```python
from build123d import *

# Parameters (mm, degrees)
F1_DEPTH  = 63.5
F0_W      = 25.4
F0_H      = 5.545384808
F0_H_2    = 19.05
F0_H_3    = 3.979615192
F2_DEPTH  = 17.526
F3_DEPTH  = 25.4
F4_DEPTH  = 7.9375
F4_FACE_W = 68.3895
F4_FACE_H = 28.575
F6_R      = 6.35


with BuildPart() as f1:
    # F0 (on Front) → F1 (new body, symmetric)
    with BuildSketch(Plane.XZ):
        Polygon((-41.275, -9.525), (41.275, -9.525), (41.275, 9.525), (22.225, 9.525), (-41.275, 9.525), align=None)
    extrude(amount=F1_DEPTH, both=True)

    # F0 (on Front) → F2 (join, symmetric)
    with BuildSketch(Plane.XZ):
        Polygon((-41.275, -9.525), (41.275, -9.525), (41.275, 9.525), (22.225, 9.525), (-41.275, 9.525), align=None)
        with BuildLine():
            Line((22.225, 9.525), (41.275, 9.525))
            Line((41.275, 9.525), (41.275, 28.8728918047))
            ThreePointArc((41.275, 28.8728918047), (44.1836383767, 35.8949660218), (51.2057125939, 38.8036043985))
            Line((51.2057125939, 38.8036043985), (60.325, 38.8036043985))
            Line((60.325, 38.8036043985), (60.325, 57.8536043985))
            Line((60.325, 57.8536043985), (51.2057125939, 57.8536043985))
            ThreePointArc((51.2057125939, 57.8536043985), (30.7132541951, 49.3653502034), (22.225, 28.8728918047))
            Line((22.225, 28.8728918047), (22.225, 9.525))
        make_face()
        with BuildLine():
            add(Edge.make_bspline(
                [(-41.275, 9.525), (-35.7294939458, 54.0499053895), (8.4615461528, 64.4009560347), (60.325, 63.3989892066)],
                knots=[0, 0, 0, 0, 114.9998552739, 114.9998552739, 114.9998552739, 114.9998552739], degree=3))
            Line((-41.275, 9.525), (22.225, 9.525))
            Line((22.225, 9.525), (22.225, 28.8728918047))
            ThreePointArc((22.225, 28.8728918047), (30.7132541951, 49.3653502034), (51.2057125939, 57.8536043985))
            Line((51.2057125939, 57.8536043985), (60.325, 57.8536043985))
            Line((60.325, 57.8536043985), (60.325, 63.3989892066))
        make_face()
        with Locations((73.025, 60.6262968025)):
            Rectangle(F0_W, F0_H)
        Polygon((111.125, 63.3989892066), (85.725, 63.3989892066), (85.725, 57.8536043985), (85.725, 38.8036043985), (85.725, 34.8239892066), (111.125, 34.8239892066), align=None)
        with Locations((73.025, 48.3286043985)):
            Rectangle(F0_W, F0_H_2)
        with Locations((73.025, 36.8137968025)):
            Rectangle(F0_W, F0_H_3)
    extrude(amount=F2_DEPTH, both=True)

    # F3 (add, symmetric): a face of the model
    f3_faces = [f1.faces().sort_by_distance(p)[0] for p in [
        (31.3502124895, -17.526, 38.5126856462),
    ]]
    extrude(f3_faces, amount=F3_DEPTH, both=True)

    # F4 (add, symmetric): a face of the model
    f4_faces = [f1.faces().sort_by_distance(p)[0] for p in [
        (31.3502124895, -42.926, 38.5126856462),
    ]]
    extrude(f4_faces, amount=F4_DEPTH, both=True)

    # F4_face (on face) → F5 (revolve)
    with BuildSketch(Plane(origin=(111.125, -16.66875, 49.1114892066), x_dir=(0, 1, 0), z_dir=(1, 0, 0))):
        Rectangle(F4_FACE_W, F4_FACE_H)
    revolve(axis=Axis((111.125, -50.8635, 49.1114892066), (0, 0, 1)))

    # F6
    f6_edges = [f1.edges().sort_by_distance(p)[0] for p in [
        (-41.275, -63.5, 0),
        (41.275, -63.5, 0),
        (41.275, 63.5, 0),
        (-41.275, 63.5, 0),
    ]]
    fillet(f6_edges, radius=F6_R)


solid = f1.part
```
CAD build for the part. Positions are in the model's coordinates, mm. A direction names the side the tool comes from. Round coordinates to 2 decimals unless told otherwise and drop trailing zeros. Write each loop counter-clockwise with the first axis right and the second up, starting at its lowest first coordinate (ties: lowest second). Pieces come first, ordered by that corner, then holes.
Item 1: Mould opens along X. For faces 5 (the cylindrical face through (43.01, -9.55, 34.48)), 6 (the cylindrical face through (39.464, -61.59, 0.133)), 7 (the flat face through (0, -63.5, 0)), 8 (the cylindrical face through (51.125, -18.043, 36.399)) say: released by +X, released by -X, zero draft, split by the parting line, or undercut.
Filled in:
face 5: undercut
face 6: released by +X
face 7: zero draft
face 8: undercut
Item 2: Band-saw the part on A-A on z = -2. Write the cut outline in (x, y) (3 decimals).
Filled in:
outline: (-41.275, -57.15) arc R6.35 ccw to (-34.925, -63.5) - (34.925, -63.5) arc R6.35 ccw to (41.275, -57.15) - (41.275, 57.15) arc R6.35 ccw to (34.925, 63.5) - (-34.925, 63.5) arc R6.35 ccw to (-41.275, 57.15) - close
Item 3: Band-saw the part on C-C on x = 71. Write the cut outline in (y, z), then the cut area to 3 significant figures.
Filled in:
outline: (-106.24, 34.82) - (17.53, 34.82) - (17.53, 63.4) - (-106.24, 63.4) - close
area: 3,540 mm2
Item 4: Band-saw the part on B-B on y = 25.5. Write the cut outline in (x, z) (3 decimals), then the cut area to 3 significant figures.
Filled in:
outline: (-41.275, -9.525) - (41.275, -9.525) - (41.275, 9.525) - (-41.275, 9.525) - close
area: 1,570 mm2
Item 5: Drop flat-ended pins along their axis: pin 1 Ø10 at (y, z) = (-46, 22) entering from -X; pin 2 Ø10 at (x, y) = (54, -3) entering from -Z; pin 3 Ø3 at (y, z) = (11, 55.5) entering from -X. Give the stop position or say it passes through.
Filled in:
pin 1: stops at x = -39.91
pin 2: stops at z = 38.56
pin 3: stops at x = -6.77
Item 6: Drill centre lines: L1, parallel to Z at x = 165, y = -72; L2, parallel to X at y = -28.5, z = 35.5; L3, parallel to Y at x = 17.5, z = 49. Where is each one in solid material? Low to high.
Filled in:
L1: z = 34.82 to 63.4
L2: x = -31.4 to 43.81, 46.5 to 175.75
L3: y = -50.86 to 17.53
Item 7: Tool access for faces 1 (the flat face through (34, 17.526, 37)), 2 (the flat face through (56, 4, 38.804)), 3 (the flat face through (1, -57, 9.525)), 4 (the flat face through (110, -50, 34.824)): list every direction of +Z, -Z, +X, -X, +Y, -Y with a clear straight run to the whole face (end or side of a thin tool).
Filled in:
face 1: +Z, +X, -X, +Y
face 2: -Z, +Y
face 3: +Z, +X, -X, -Y
face 4: -Z, +X, +Y, -Y
